Geometry: final body of the model. Coordinates: model frame, mm. A direction names the side the tool comes from. Round coordinates to 2 decimals unless told otherwise and drop trailing zeros. Write each loop counter-clockwise with the first axis right and the second up, starting at its lowest first coordinate (ties: lowest second). Pieces come first, ordered by that corner, then holes. Notation, with made-up numbers: (85, -28) -> (143, -28) arc R11 cw to (143, -10) -> close; hole circle Ø6 at (39.5, 39.25). An arc over 180 degrees is marked (long way). One line per item, written item: value. Start each with the question number.
from build123d import *

# Parameters (mm, degrees)
BOSS_EXTRUDE1_DEPTH     = 5
SKETCH2_W               = 5
SKETCH2_H               = 64.125
BOSS_EXTRUDE2_DEPTH     = 25
CUT_EXTRUDE1_DEPTH      = 173.980490229
CUT_EXTRUDE1_DEPTH_BACK = 173.980490229
SKETCH3_R               = 2.5
CUT_EXTRUDE2_DEPTH      = 139.496389845
CUT_EXTRUDE2_DEPTH_BACK = 139.496389845
SKETCH4_R               = 2.5


with BuildPart() as part:
    # Sketch1 → Boss-Extrude1 (new body)
    with BuildSketch(Plane(origin=(0, 0, 0), x_dir=(1, 0, 0), z_dir=(0, 1, 0))):
        with BuildLine():
            Line((-75, 15.75), (-75, -15.75))
            Line((-75, -15.75), (-54, -15.75))
            Line((-54, -15.75), (-54, -79.875))
            Line((-54, -79.875), (-70.25200942, -79.875))
            ThreePointArc((-70.25200942, -79.875), (-72.104159031, -81.120320055), (-71.649789587, -83.305458181))
            ThreePointArc((-71.649789587, -83.305458181), (0, -112.5), (71.649789587, -83.305458181))
            ThreePointArc((71.649789587, -83.305458181), (72.104159031, -81.120320055), (70.25200942, -79.875))
            Line((70.25200942, -79.875), (54, -79.875))
            Line((54, -79.875), (54, -15.75))
            Line((54, -15.75), (75, -15.75))
            Line((75, -15.75), (75, 0))
            Line((75, 0), (75, 15.75))
            Line((75, 15.75), (54, 15.75))
            Line((54, 15.75), (54, 79.875))
            Line((54, 79.875), (70.25200942, 79.875))
            ThreePointArc((70.25200942, 79.875), (72.104159031, 81.120320055), (71.649789587, 83.305458181))
            ThreePointArc((71.649789587, 83.305458181), (0, 112.5), (-71.649789587, 83.305458181))
            ThreePointArc((-71.649789587, 83.305458181), (-72.104159031, 81.120320055), (-70.25200942, 79.875))
            Line((-70.25200942, 79.875), (-54, 79.875))
            Line((-54, 79.875), (-54, 15.75))
            Line((-54, 15.75), (-75, 15.75))
        make_face()
    extrude(amount=BOSS_EXTRUDE1_DEPTH)

    # Sketch2 → Boss-Extrude2 (add)
    with BuildSketch(Plane.XZ):
        with Locations((51.5, 47.8125)):
            Rectangle(SKETCH2_W, SKETCH2_H)
        with Locations((-51.5, 47.8125)):
            Rectangle(SKETCH2_W, SKETCH2_H)
        with Locations((-51.5, -47.8125)):
            Rectangle(SKETCH2_W, SKETCH2_H)
        with Locations((51.5, -47.8125)):
            Rectangle(SKETCH2_W, SKETCH2_H)
    extrude(amount=BOSS_EXTRUDE2_DEPTH)

    # Sketch3 → Cut-Extrude1 (cut, two sides: drawn at the far end of the back side and taken through both)
    with BuildSketch(Plane(origin=(54, 0, 0), x_dir=(0, 0, -1), z_dir=(1, 0, 0)).offset(-CUT_EXTRUDE1_DEPTH_BACK)):
        with Locations(Location((-47.8125, -12.36, 0), (0, 0, 180))):
            Circle(SKETCH3_R)
        with Locations((47.8125, -12.36)):
            Circle(SKETCH3_R)
    extrude(amount=CUT_EXTRUDE1_DEPTH + CUT_EXTRUDE1_DEPTH_BACK, mode=Mode.SUBTRACT)

    # Sketch4 → Cut-Extrude2 (cut, two sides: drawn at the far end of the back side and taken through both)
    with BuildSketch(Plane(origin=(0, 5, 0), x_dir=(1, 0, 0), z_dir=(0, 1, 0)).offset(-CUT_EXTRUDE2_DEPTH_BACK)):
        with Locations(Location((-62.5, 85, 0), (0, 0, 270))):
            Circle(SKETCH4_R)
        with Locations(Location((62.5, 85, 0), (0, 0, 270))):
            Circle(SKETCH4_R)
        with Locations(Location((62.5, 0, 0), (0, 0, 270))):
            Circle(SKETCH4_R)
        with Locations(Location((62.5, -85, 0), (0, 0, 270))):
            Circle(SKETCH4_R)
        with Locations(Location((-62.5, 0, 0), (0, 0, 270))):
            Circle(SKETCH4_R)
        with Locations(Location((-62.5, -85, 0), (0, 0, 270))):
            Circle(SKETCH4_R)
    extrude(amount=CUT_EXTRUDE2_DEPTH + CUT_EXTRUDE2_DEPTH_BACK, mode=Mode.SUBTRACT)


solid = part.part
(1) Line query: probe 1 along X at (y, z) = (-4.25, 74); probe 2 along X at (y, z) = (3, 85); probe 3 along Y at (x, z) = (19.5, 42). Output: solid intervals per line, ascending.
(2) Section query A-A (y = -12.36). Count the separate pieces of the cut face and the enclosed holes in it, and give its area (3 significant figures).
(3) Pin query (flat end, axial travel): pin 1 (7.5 mm diameter, centred on y = -16, z = -45.5, fed in from +X); pin 2 (6.5 mm diameter, centred on x = 62.5, z = 0, fed in from -Y); pin 3 (5.5 mm diameter, centred on x = 51, y = -16, fed in from -Z) (3 decimals). Return the tip coordinate at first contact, or that it passes through.
(4) Section query B-B (z = 0). Output: boundary loops of the cut face in (x, y).
(5) Pull-direction query (Z, two-part tool) for faces 4 (the face through (-75, 2, 0)), 5 (the face through (-52, -12, 79.875)), 6 (the face through (51.46, -13.32, -50.12)); classes: pulls with the +Z half, pulls with the -Z half, needs draft (parallel to the pull), parting line crosses it, or undercut.
(6) Section query D-D (z = 62). Output: boundary loops of the cut face in (x, y), and give its area (3 significant figures).
(7) Set-up query: faces 1 (the face through (-49, -9.5, 47.4)), 2 (the face through (-52, -12, -15.75)), 3 (the face through (62, 2, -79.875)). Return all of +Z, -Z, +X, -X, +Y, -Y with unobstructed straight access to the full face (end or side cutting, diameter ignored); none if empty.
(8) Section query C-C (x = -62.5). Output: boundary loops of the cut face in (y, z) (3 decimals).
Results list:
1. probe 1: x = -54 to -49, 49 to 54
1. probe 2: x = -69.87 to -65, -60 to 60, 65 to 69.87
1. probe 3: y = 0 to 5
2. separate pieces: 8
2. enclosed holes: 0
2. area: 1,180 mm^2
3. pin 1: stops at x = 54
3. pin 2: stops at y = 0
3. pin 3: stops at z = -79.875
4. outline: (-75, 0) -> (-65, 0) -> (-65, 5) -> (-75, 5) -> close; (-60, 0) -> (60, 0) -> (60, 5) -> (-60, 5) -> close; (65, 0) -> (75, 0) -> (75, 5) -> (65, 5) -> close
5. face 4: needs draft
5. face 5: pulls with the +Z half
5. face 6: undercut
6. outline: (-54, -25) -> (-49, -25) -> (-49, 0) -> (49, 0) -> (49, -25) -> (54, -25) -> (54, 5) -> (-54, 5) -> close
6. area: 790 mm^2
7. face 1: +Z, -Z, -Y
7. face 2: +X, -X, -Y
7. face 3: +X, +Y, -Y
8. outline: (0, -91.245) -> (5, -91.245) -> (5, -87.5) -> (0, -87.5) -> close; (0, -82.5) -> (5, -82.5) -> (5, -79.875) -> (0, -79.875) -> close; (0, -15.75) -> (5, -15.75) -> (5, -2.5) -> (0, -2.5) -> close; (0, 2.5) -> (5, 2.5) -> (5, 15.75) -> (0, 15.75) -> close; (0, 79.875) -> (5, 79.875) -> (5, 82.5) -> (0, 82.5) -> close; (0, 87.5) -> (5, 87.5) -> (5, 91.245) -> (0, 91.245) -> close
